Check sheet for the modelled part. Datum: model origin and axes. Units: mm. Give positions to 0.01 mm unless a question says otherwise; leave off trailing zeros. Write each loop counter-clockwise with the first axis right and the second up, starting at its lowest first coordinate (ties: lowest second). Pieces come first, ordered by that corner, then holes. Notation, with made-up numbers: M 42.5,-34.75 L 78.5,-34.75 A28 ccw 78.5,-7.75 Z; hole C 55,53 d10. An arc over 180 degrees is marked long. Write item = value, one per line. Start each with the question number.
1) Cross-section at A-A, the plane z = 0. Record the cut outline in (x, y).
2) Cross-section at B-B, the plane y = 1.1. Record the cut outline in (x, z), plus the area to 3 significant figures.
3) Go/stop test with a flat-tipped pin: pin 1 (3 mm diameter, centred on x = -26.75, z = 0, fed in from -Y). Record where the tip stops, or that it passes through.
4) Scan lines: line 1 along X through (y, z) = (0.7, 0); line 2 along X through (y, z) = (0.6, -1.25); line 3 along Z through (x, y) = (-26.75, 1.4). Record each from-to range of solid material in increasing order. Write a range as [from, to].
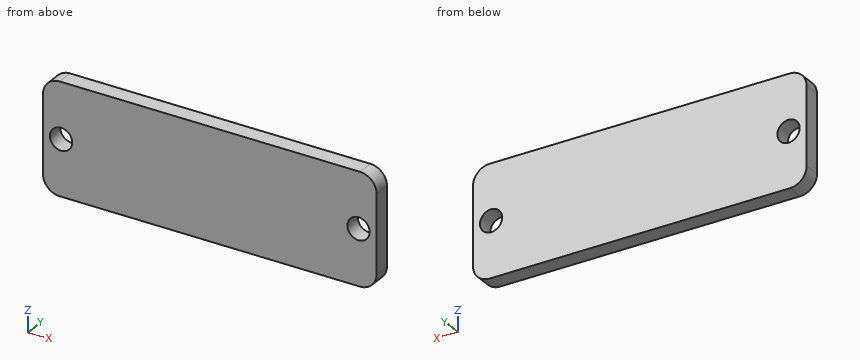
```python
from build123d import *

# Parameters (mm, degrees)
SKETCH_1_W          = 60
SKETCH_1_H          = 20
EXTRUDE_1_DEPTH     = 3
FILLET_1_R          = 3
SKETCH_2_R          = 2
CUT_EXTRUDE_1_DEPTH = 3


with BuildPart() as part:
    # Эскиз1 → Бобышка-Вытянуть1 (new body)
    with BuildSketch(Plane(origin=(0, 0, 0), x_dir=(1, 0, 0), z_dir=(0, 1, 0))):
        Rectangle(SKETCH_1_W, SKETCH_1_H)
    extrude(amount=EXTRUDE_1_DEPTH)

    # Скругление1
    fillet_1_edges = [part.edges().sort_by_distance(p)[0] for p in [
        (30, 1.5, 10),
        (-30, 1.5, 10),
        (-30, 1.5, -10),
        (30, 1.5, -10),
    ]]
    fillet(fillet_1_edges, radius=FILLET_1_R)

    # Эскиз2 → Вырез-Вытянуть1 (cut)
    with BuildSketch(Plane(origin=(0, 3, 0), x_dir=(1, 0, 0), z_dir=(0, 1, 0))):
        with Locations(Location((26.75, 0, 0), (0, 0, 270))):
            Circle(SKETCH_2_R)
        with Locations(Location((-26.75, 0, 0), (0, 0, 90))):
            Circle(SKETCH_2_R)
    extrude(amount=-CUT_EXTRUDE_1_DEPTH, mode=Mode.SUBTRACT)


solid = part.part
```
Reply:
q1.outline = M -30,0 L -28.75,0 L -28.75,3 L -30,3 Z; M -24.75,0 L 24.75,0 L 24.75,3 L -24.75,3 Z; M 28.75,0 L 30,0 L 30,3 L 28.75,3 Z
q2.outline = M -30,-7 A3 ccw -27,-10 L 27,-10 A3 ccw 30,-7 L 30,7 A3 ccw 27,10 L -27,10 A3 ccw -30,7 Z; hole C -26.75,0 d4; hole C 26.75,0 d4
q2.area = 1,170 mm2
q3.pin_1 = through
q4.line_1 = [-30, -28.75], [-24.75, 24.75], [28.75, 30]
q4.line_2 = [-30, -28.31], [-25.19, 25.19], [28.31, 30]
q4.line_3 = [-10, -2], [2, 10]
